Verification items for the finished model (mm, model axes). Coordinates: 2 decimals unless noted, no trailing zeros. Loops run counter-clockwise (first coordinate to the right, second up) from the corner with the lowest first, then second, coordinate; pieces in that order, holes last. Notation, with made-up numbers: (85.25, -36.5) -> (114.25, -36.5) arc R16 ccw to (114.25, -12.5) -> close; hole circle Ø4 at (-19.75, 36). An arc over 180 degrees is marked (long way). Write item = value, one per line.
Autodesk Inventor part; units mm, degrees
ref_plane "Plano de trabajo1" through (0, 0, -308.9) normal (0, 0, 1) x (1, 0, 0)
ref_plane "YZ Plane" through (0, 0, 0) normal (1, 0, 0) x (0, 1, 0)
ref_plane "XZ Plane" through (0, 0, 0) normal (0, 1, 0) x (-1, 0, 0)
sketch "Boceto1" plane through (0, 0, 0) normal (0, 0, 1) x (1, 0, 0)
  line L0 (28.5, 53.7) -> (28.5, 47.2)
  line L1 (26.1, 47.2) -> (28.5, 47.2)
  line L2 (26.1, 48.45) -> (25.3942, 48.45)
  line L3 (25.3942, 48.45) -> (24.7, 47.44)
  line L4 (26.1, 52.45) -> (25.3942, 52.45)
  line L5 (26.1, 53.7) -> (28.5, 53.7)
  line L6 (24.7, 53.46) -> (25.3942, 52.45)
  line L7 (26.1, 53.7) -> (26.1, 52.45)
  line L8 (26.1, 47.2) -> (26.1, 48.45)
  line L9 (21.2, 47.44) -> (24.7, 47.44)
  line L10 (21.2, 53.46) -> (21.2, 47.44)
  line L11 (21.2, 53.46) -> (24.7, 53.46)
  point P0 (28.5, 50.45)
  dimension "d78" = 6.5
  dimension "d88" = 2.4
  dimension "d95" = 6.02
  dimension "d100" = 2.4
  dimension "d108" = 4
  dimension "d109" = 0.7058
  dimension "d110" = 0.7058
  dimension "d145" = 2
  dimension "d146" = 2
  dimension "d150" = 3.5
  dimension "d151" = 3.5
extrude "Extrusión1" add sketch "Boceto1" against normal blind 617.8
ref_plane "Plano de trabajo1" through (0, 0, -308.9) normal (0, 0, 1) x (1, 0, 0)
sketch "Boceto2" plane through (28.5, -22.9, 0) normal (-1, 0, 0) x (0, 0, 1)
  line L0 (-617.8, 76.6) -> (-617.8, 70.1)
  line L1 (-617.8, 70.1) -> (-617.8, 76.6)
  line L2 (-617.8, 76.6) -> (-611.3, 76.6)
  line L3 (0, 76.6) -> (-617.8, 76.6)
  line L4 (-617.8, 70.1) -> (-611.3, 76.6)
  dimension "d149" = 45
extrude "Extrusión2" cut sketch "Boceto2" along normal through all
mirror "Simetría1" about plane through (0, 0, -308.9) normal (0, 0, 1) of "Extrusión2"
properties part number "SP40-02 JUNTA INT 207" material "Caucho, negro"
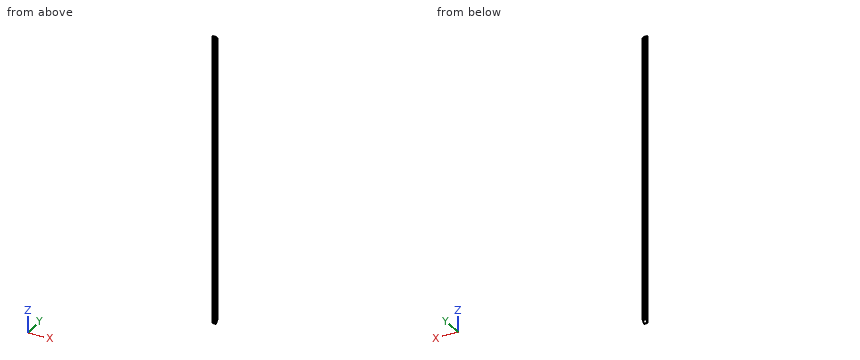
1) Material ranges on line 1 (Y direction, x = 23.75, z = -142); line 2 (X direction, y = 52.5, z = -355.5); line 3 (Y direction, x = 25.5, z = -532), recorded low to high.
Ans:
line_1 = 47.44 to 53.46
line_2 = 21.2 to 25.36, 26.1 to 28.5
line_3 = 48.45 to 52.45
2) Depth check by flat-ended pin: pin 1 Ø4 at (x, z) = (23.5, -436) entering from +Y; pin 2 Ø3 at (x, y) = (23, 52.5) entering from +Z; pin 3 Ø3 at (x, z) = (23, -324) entering from -Y. Enter the tip coordinate at first touch or a pass-through.
Ans:
pin_1 = 53.46
pin_2 = -3.8
pin_3 = 47.44
3) Sectioned sample at B-B, the plane x = 23.5. Record the cut outline in (y, z).
Ans:
outline = (47.44, -617.56) -> (53.46, -611.54) -> (53.46, -6.26) -> (47.44, -0.24) -> close
4) Sectioned sample at A-A, the plane z = -472. Record the cut outline in (x, y), plus the area to 3 significant figures.
Ans:
outline = (21.2, 47.44) -> (24.7, 47.44) -> (25.39, 48.45) -> (26.1, 48.45) -> (26.1, 47.2) -> (28.5, 47.2) -> (28.5, 53.7) -> (26.1, 53.7) -> (26.1, 52.45) -> (25.39, 52.45) -> (24.7, 53.46) -> (21.2, 53.46) -> close
area = 43.0 mm2
